Model file for the job. Use its own axes, mm. Face numbers are marked on the shaded views. Round coordinates to 2 decimals unless told otherwise and drop trailing zeros. Write each loop counter-clockwise with the first axis right and the second up, starting at its lowest first coordinate (ties: lowest second). Pieces come first, ordered by that corner, then holes.
```python
from build123d import *

# Parameters (mm, degrees)
RESSALTO_EXTRUS_O1_DEPTH = 22.5
CHANFRO1_SIZE            = 10
CORTE_EXTRUS_O1_REACH    = 380.591
ESBO_O3_W                = 1139.230904301
ESBO_O3_H                = 709.798033895
CORTE_EXTRUS_O5_DEPTH    = 1.5


with BuildPart() as part:
    # Esboço1 → Ressalto-extrusão1 (new, symmetric)
    with BuildSketch(Plane.XY):
        with BuildLine():
            Line((-45, 0), (45, 0))
            ThreePointArc((45, 0), (52.071067812, 2.928932188), (55, 10))
            Line((55, 10), (55, 130))
            ThreePointArc((55, 130), (56.339745962, 135), (60, 138.660254038))
            Line((60, 138.660254038), (110, 167.527767497))
            ThreePointArc((110, 167.527767497), (113.660254038, 171.188021535), (115, 176.188021535))
            Line((115, 176.188021535), (115, 350))
            ThreePointArc((115, 350), (112.071067812, 357.071067812), (105, 360))
            Line((105, 360), (-105, 360))
            ThreePointArc((-105, 360), (-112.071067812, 357.071067812), (-115, 350))
            Line((-115, 350), (-115, 176.188021535))
            ThreePointArc((-115, 176.188021535), (-113.660254038, 171.188021535), (-110, 167.527767497))
            Line((-110, 167.527767497), (-60, 138.660254038))
            ThreePointArc((-60, 138.660254038), (-56.339745962, 135), (-55, 130))
            Line((-55, 130), (-55, 10))
            ThreePointArc((-55, 10), (-52.071067812, 2.928932188), (-45, 0))
        make_face()
        Polygon((-35, 20), (35, 20), (35, 147.320508076), (95, 181.961524227), (95, 340), (-95, 340), (-95, 181.961524227), (-35, 147.320508076), align=None, mode=Mode.SUBTRACT)
    extrude(amount=RESSALTO_EXTRUS_O1_DEPTH, both=True)

    # Chanfro1
    chanfro1_edges = [part.edges().sort_by_distance(p)[0] for p in [
        (113.660254038, 171.188021535, 22.5),
        (115, 263.094010768, 22.5),
        (115, 263.094010768, -22.5),
        (113.660254038, 171.188021535, -22.5),
        (85, 153.094010768, -22.5),
        (56.339745962, 135, -22.5),
        (55, 70, -22.5),
        (52.071067812, 2.928932188, -22.5),
        (0, 0, -22.5),
        (-52.071067812, 2.928932188, -22.5),
        (-55, 70, -22.5),
        (-56.339745962, 135, -22.5),
        (-85, 153.094010768, -22.5),
        (-113.660254038, 171.188021535, -22.5),
        (-115, 263.094010768, -22.5),
        (-112.071067812, 357.071067812, -22.5),
        (0, 360, -22.5),
        (112.071067812, 357.071067812, -22.5),
        (112.071067812, 357.071067812, 22.5),
        (0, 360, 22.5),
        (-112.071067812, 357.071067812, 22.5),
        (-115, 263.094010768, 22.5),
        (-113.660254038, 171.188021535, 22.5),
        (-85, 153.094010768, 22.5),
        (-56.339745962, 135, 22.5),
        (-55, 70, 22.5),
        (-52.071067812, 2.928932188, 22.5),
        (0, 0, 22.5),
        (52.071067812, 2.928932188, 22.5),
        (55, 70, 22.5),
        (56.339745962, 135, 22.5),
        (85, 153.094010768, 22.5),
    ]]
    chamfer(chanfro1_edges, length=CHANFRO1_SIZE - 0.0001)  # a hair under: the kernel refuses the full size

    # Esboço3 → Corte-extrusão1 (cut, up to next)
    with BuildSketch(Plane.XY, mode=Mode.PRIVATE) as corte_extrus_o1_sk1:
        with Locations((-153.157436203, 152.53565808)):
            Rectangle(ESBO_O3_W, ESBO_O3_H)
    corte_extrus_o1_tool1 = extrude(corte_extrus_o1_sk1.sketch, amount=-CORTE_EXTRUS_O1_REACH, mode=Mode.PRIVATE) & part.part
    add(corte_extrus_o1_tool1.solids().sort_by_distance((-153.157436, 152.535658, 0))[0], mode=Mode.SUBTRACT)

    # Esboço4 → Corte-extrusão5 (cut)
    with BuildSketch(Plane.XY.offset(22.5)):
        Polygon((104, 349), (-104, 349), (-104, 176.765371804), (-44, 142.124355653), (-44, 11), (44, 11), (44, 142.124355653), (104, 176.765371804), align=None)
        Polygon((-95, 340), (-95, 181.961524227), (-35, 147.320508076), (-35, 20), (0, 20), (35, 20), (35, 147.320508076), (95, 181.961524227), (95, 340), align=None, mode=Mode.SUBTRACT)
    extrude(amount=-CORTE_EXTRUS_O5_DEPTH, mode=Mode.SUBTRACT)


solid = part.part
```
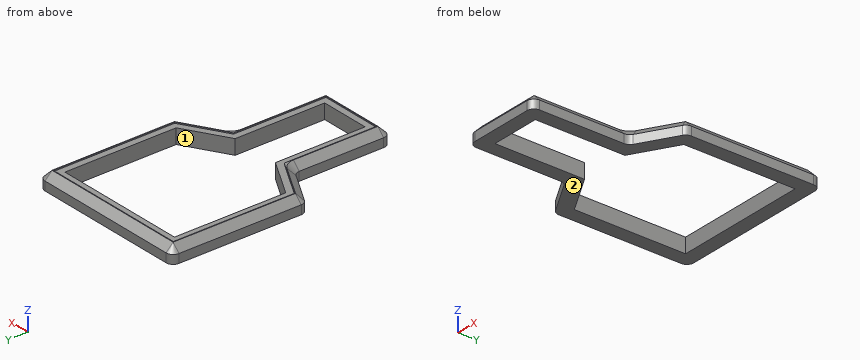
1) Cut at B-B on z = 6.75. List the corners of the cut face in (x, y).
2) Cut at A-A on y = 33. List the corners of the cut face in (x, z), and give its area (3 significant figures).
3) Pull direction X, two halves, no side cores. Call the marked faces 1 and 2: released by +X, released by -X, zero draft, split by the parting line, or undercut.
4) Flat gauge pins, fed straight in: pin 1 Ø8 at (x, y) = (33.5, 153) entering from +Z; pin 2 Ø1.6 at (x, z) = (-46, 22) entering from -Y; pin 3 Ø3 at (x, z) = (68, 15) entering from -Y; pin 4 Ø1.6 at (y, z) = (106, 21.5) entering from -X. Where does each tip first touch, or does it go through?
5) Wall check: probe 1 along X at (y, z) = (115, 9.25); probe 2 along X at (y, z) = (249.5, 12); probe 3 along Y at (x, z) = (-57, 19.5). Give the ranges that are in metal, low to high.
6) Cut at C-C on x = 14. List the corners of the cut face in (y, z), and give its area (3 significant figures).
Result sheet:
1. outline: (-115, 176.19) arc R10 ccw to (-110, 167.53) - (-60, 138.66) arc R10 cw to (-55, 130) - (-55, 10) arc R10 ccw to (-45, 0) - (45, 0) arc R10 ccw to (55, 10) - (55, 130) arc R10 cw to (60, 138.66) - (110, 167.53) arc R10 ccw to (115, 176.19) - (115, 350) arc R10 ccw to (105, 360) - (-105, 360) arc R10 ccw to (-115, 350) - close; hole (-95, 181.96) - (-35, 147.32) - (-35, 20) - (35, 20) - (35, 147.32) - (95, 181.96) - (95, 340) - (-95, 340) - close
2. outline: (-55, 0) - (-35, 0) - (-35, 21) - (-44, 21) - (-44, 22.5) - (-45, 22.5) - (-55, 12.5) - close; (35, 0) - (55, 0) - (55, 12.5) - (45, 22.5) - (44, 22.5) - (44, 21) - (35, 21) - close
2. area: 773 mm2
3. face 1: undercut
3. face 2: zero draft
4. pin 1: passes through
4. pin 2: stops at y = 8.97
4. pin 3: stops at y = 144.23
4. pin 4: stops at x = -46.8
5. probe 1: x = -55 to -35, 35 to 55
5. probe 2: x = -115 to -95, 95 to 115
5. probe 3: y = 145.01 to 160.02, 340 to 353
6. outline: (0, 0) - (20, 0) - (20, 21) - (11, 21) - (11, 22.5) - (10, 22.5) - (0, 12.5) - close; (340, 0) - (360, 0) - (360, 12.5) - (350, 22.5) - (349, 22.5) - (349, 21) - (340, 21) - close
6. area: 773 mm2
